from build123d import *

# Parameters (mm, degrees)
SKETCH1_W           = 220
SKETCH1_H           = 180
BOSS_EXTRUDE1_DEPTH = 45
FILLET1_R           = 5
CUT_EXTRUDE7_DEPTH  = 42
CUT_EXTRUDE2_DEPTH  = 5
CUT_EXTRUDE3_DEPTH  = 5
SKETCH4_W           = 11.5
SKETCH4_H           = 6.5
CUT_EXTRUDE4_DEPTH  = 5
SKETCH5_W           = 45.536818034
SKETCH5_H           = 10
CUT_EXTRUDE5_DEPTH  = 5
SKETCH6_W           = 18
SKETCH6_H           = 8.5
CUT_EXTRUDE6_DEPTH  = 5
SKETCH8_W           = 5
SKETCH8_H           = 9
CUT_EXTRUDE8_DEPTH  = 4.2
SKETCH10_R          = 2.5
CUT_EXTRUDE9_DEPTH  = 40


with BuildPart() as part:
    # Sketch1 → Boss-Extrude1 (new body)
    with BuildSketch(Plane(origin=(0, 0, 0), x_dir=(1, 0, 0), z_dir=(0, 1, 0))):
        with Locations((110, 90)):
            Rectangle(SKETCH1_W, SKETCH1_H)
    extrude(amount=BOSS_EXTRUDE1_DEPTH)

    # Fillet1
    fillet1_edges = [part.edges().sort_by_distance(p)[0] for p in [
        (0, 22.5, -180),
        (220, 22.5, -180),
        (220, 22.5, 0),
        (0, 22.5, 0),
    ]]
    fillet(fillet1_edges, radius=FILLET1_R)

    # Sketch7 → Cut-Extrude7 (cut)
    with BuildSketch(Plane(origin=(0, 45, 0), x_dir=(1, 0, 0), z_dir=(0, 1, 0))):
        with BuildLine():
            Line((207, 177), (13, 177))
            ThreePointArc((13, 177), (10.071067812, 169.928932188), (3, 167))
            Line((3, 167), (3, 13))
            ThreePointArc((3, 13), (10.071067812, 10.071067812), (13, 3))
            Line((13, 3), (207, 3))
            ThreePointArc((207, 3), (209.928932188, 10.071067812), (217, 13))
            Line((217, 13), (217, 167))
            ThreePointArc((217, 167), (209.928932188, 169.928932188), (207, 177))
        make_face()
    extrude(amount=-CUT_EXTRUDE7_DEPTH, mode=Mode.SUBTRACT)

    # Sketch2 → Cut-Extrude2 (cut)
    with BuildSketch(Plane.XY):
        Polygon((175.9, 35), (178.4, 35), (180, 33.4), (180, 24.5), (174.3, 24.5), (174.3, 33.4), align=None)
        Polygon((190.9, 35), (193.4, 35), (195, 33.4), (195, 24.5), (189.3, 24.5), (189.3, 33.4), align=None)
        Polygon((160.9, 35), (163.4, 35), (165, 33.4), (165, 24.5), (159.3, 24.5), (159.3, 33.4), align=None)
        Polygon((145.9, 35), (148.4, 35), (150, 33.4), (150, 24.5), (144.3, 24.5), (144.3, 33.4), align=None)
        Polygon((130.9, 35), (133.4, 35), (135, 33.4), (135, 24.5), (129.3, 24.5), (129.3, 33.4), align=None)
        Polygon((115.9, 35), (118.4, 35), (120, 33.4), (120, 24.5), (114.3, 24.5), (114.3, 33.4), align=None)
        Polygon((100.9, 35), (103.4, 35), (105, 33.4), (105, 24.5), (99.3, 24.5), (99.3, 33.4), align=None)
        Polygon((85.9, 35), (88.4, 35), (90, 33.4), (90, 24.5), (84.3, 24.5), (84.3, 33.4), align=None)
    extrude(amount=-CUT_EXTRUDE2_DEPTH, mode=Mode.SUBTRACT)

    # Sketch3 → Cut-Extrude3 (cut)
    with BuildSketch(Plane.XY):
        Polygon((22.5, 32.9), (36, 32.9), (36, 24.5), (22.5, 24.5), (20, 27), (20, 30.4), align=None)
    extrude(amount=-CUT_EXTRUDE3_DEPTH, mode=Mode.SUBTRACT)

    # Sketch4 → Cut-Extrude4 (cut)
    with BuildSketch(Plane.XY):
        with Locations((51.75, 28.75)):
            Rectangle(SKETCH4_W, SKETCH4_H)
        with Locations((68.55, 28.75)):
            Rectangle(SKETCH4_W, SKETCH4_H)
    extrude(amount=-CUT_EXTRUDE4_DEPTH, mode=Mode.SUBTRACT)

    # Sketch5 → Cut-Extrude5 (cut)
    with BuildSketch(Plane(origin=(220, 0, 0), x_dir=(0, 0, -1), z_dir=(1, 0, 0))):
        with Locations((90, 19.480228536)):
            Rectangle(SKETCH5_W, SKETCH5_H)
    extrude(amount=-CUT_EXTRUDE5_DEPTH, mode=Mode.SUBTRACT)

    # Sketch6 → Cut-Extrude6 (cut)
    with BuildSketch(Plane(origin=(0, 0, -180), x_dir=(-1, 0, 0), z_dir=(0, 0, -1))):
        with Locations((-193, 19.25)):
            Rectangle(SKETCH6_W, SKETCH6_H)
        with Locations((-170, 19.25)):
            Rectangle(SKETCH6_W, SKETCH6_H)
        with Locations((-147, 19.25)):
            Rectangle(SKETCH6_W, SKETCH6_H)
        with Locations((-124, 19.25)):
            Rectangle(SKETCH6_W, SKETCH6_H)
    extrude(amount=-CUT_EXTRUDE6_DEPTH, mode=Mode.SUBTRACT)

    # Sketch8 → Cut-Extrude8 (cut)
    with BuildSketch(Plane.ZY):
        with Locations((-155.038386618, 29)):
            Rectangle(SKETCH8_W, SKETCH8_H)
    extrude(amount=-CUT_EXTRUDE8_DEPTH, mode=Mode.SUBTRACT)

    # Sketch10 → Cut-Extrude9 (cut)
    with BuildSketch(Plane(origin=(0, 45, 0), x_dir=(1, 0, 0), z_dir=(0, 1, 0))):
        with Locations(Location((6.5, 173.5, 0), (0, 0, 270))):
            Circle(SKETCH10_R)
        with Locations(Location((213.5, 173.5, 0), (0, 0, 90))):
            Circle(SKETCH10_R)
        with Locations(Location((213.5, 6.5, 0), (0, 0, 270))):
            Circle(SKETCH10_R)
        with Locations(Location((6.5, 6.5, 0), (0, 0, 90))):
            Circle(SKETCH10_R)
    extrude(amount=-CUT_EXTRUDE9_DEPTH, mode=Mode.SUBTRACT)


solid = part.part
Here's how the part is built. I have some questions about the finished solid (model axes, mm). A direction names the side the tool comes from. Give positions to 0.01 mm unless a question says otherwise; leave off trailing zeros. Order: outer loops, then holes, each group sorted by start corner. A loop starts at its lowest first (then second) coordinate and runs counter-clockwise, first axis right, second up. Notation, with made-up numbers: (-32.5, -35.5) -> (-19.5, -35.5) arc R17 ccw to (-19.5, -4.5) -> close; hole circle Ø3 at (8.25, 39). An arc over 180 degrees is marked (long way). Use a Markdown table: item, result. Add a question column.
Item 1: If we mould it in two halves opening along X, with no side actions, what happens to faces 3 (the face through (220, 27, -89)), 4 (the face through (0, 22, -89)), 5 (the face through (7, 5, -174))? For each: pulls with the +X half, pulls with the -X half, needs draft (parallel to the pull), parting line crosses it, or undercut.
Item 2: Will these pins go through, and if not, where does the flat tip stop? pin 1 (3 mm diameter, centred on x = 160, z = -147, fed in from +Y); pin 2 (2.5 mm diameter, centred on y = 31, z = -1, fed in from +X); pin 3 (1.5 mm diameter, centred on y = 30.5, z = -1.5, fed in from -X).
Item 3: Imagine slicing it at A-A on z = -74.5. Please give me the cut outline in (x, y), plus the area to 3 significant figures.
Item 4: For faces 1 (the face through (215.98, 25.28, -6.83)), 2 (the face through (109, 22, -180)), which set-ups out of +Z, -Z, +X, -X, +Y, -Y let a thin tool reach every point of the face, with its end or its side?
Item 5: Imagine slicing it at B-B on y = 41. Please give me the cut outline in (x, z).
Item 6: I need wall thicknesses on line 1 (X direction, y = 26, z = -162.5); line 2 (X direction, y = 15, z = -173.5); line 3 (Z direction, x = 213.5, y = 15). Which ranges of each line are inside material? Lowest first, please.
Item 7: Imagine slicing it at C-C on x = 78.5. Please give me the cut outline in (y, z), plus the area to 3 significant figures.
Item 8: Imagine slicing it at D-D on z = -119.5. Please give me the cut outline in (x, y), plus the area to 3 significant figures.
Data:
| question | item | result |
|---|---|---|
| 1 | face 3 | pulls with the +X half |
| 1 | face 4 | pulls with the -X half |
| 1 | face 5 | undercut |
| 2 | pin 1 | stops at y = 3 |
| 2 | pin 2 | stops at x = 219.18 |
| 2 | pin 3 | stops at x = 0.82 |
| 3 | outline | (0, 0) -> (220, 0) -> (220, 14.48) -> (217, 14.48) -> (217, 3) -> (3, 3) -> (3, 45) -> (0, 45) -> close; (217, 24.48) -> (220, 24.48) -> (220, 45) -> (217, 45) -> close |
| 3 | area | 882 mm² |
| 4 | face 1 | +Y |
| 4 | face 2 | -Z, +X, -X, +Y, -Y |
| 5 | outline | (0, -175) arc R5 ccw to (5, -180) -> (215, -180) arc R5 ccw to (220, -175) -> (220, -5) arc R5 ccw to (215, 0) -> (5, 0) arc R5 ccw to (0, -5) -> close; hole (3, -167) arc R10 cw to (13, -177) -> (207, -177) arc R10 cw to (217, -167) -> (217, -13) arc R10 cw to (207, -3) -> (13, -3) arc R10 cw to (3, -13) -> close; hole circle Ø5 at (6.5, -173.5); hole circle Ø5 at (6.5, -6.5); hole circle Ø5 at (213.5, -173.5); hole circle Ø5 at (213.5, -6.5) |
| 6 | line 1 | x = 0 to 3, 217 to 220 |
| 6 | line 2 | x = 0 to 4, 9 to 12.37, 207.63 to 211, 216 to 220 |
| 6 | line 3 | z = -180 to -176, -171 to -167.63, -12.37 to -9, -4 to 0 |
| 7 | outline | (0, -180) -> (45, -180) -> (45, -177) -> (3, -177) -> (3, -3) -> (45, -3) -> (45, 0) -> (0, 0) -> close |
| 7 | area | 792 mm² |
| 8 | outline | (0, 0) -> (220, 0) -> (220, 45) -> (217, 45) -> (217, 3) -> (3, 3) -> (3, 45) -> (0, 45) -> close |
| 8 | area | 912 mm² |
